```python
from build123d import *

# Parameters (mm, degrees)
SKETCH1_R           = 6
SKETCH1_R_2         = 2
BOSS_EXTRUDE1_DEPTH = 28.5
SKETCH2_R           = 2
SKETCH2_R_2         = 1
BOSS_EXTRUDE2_DEPTH = 3
SKETCH3_R           = 4
CUT_EXTRUDE1_DEPTH  = 23
SKETCH4_W           = 13
SKETCH4_H           = 13
SKETCH4_W_2         = 10
SKETCH4_H_2         = 10
CUT_EXTRUDE2_DEPTH  = 35.503622998
CUT_EXTRUDE5_DEPTH  = 33.003091855
SKETCH9_W           = 5
SKETCH9_H           = 4.708815116
CUT_EXTRUDE6_DEPTH  = 36.548469223
CUT_EXTRUDE7_DEPTH  = 35.412176554
SKETCH11_R          = 1.5
CUT_EXTRUDE8_DEPTH  = 32.929610206
FILLET1_R           = 2


with BuildPart() as part:
    # Sketch1 → Boss-Extrude1 (new body)
    with BuildSketch(Plane(origin=(0, 0, 0), x_dir=(1, 0, 0), z_dir=(0, 1, 0))):
        with Locations(Location((0, 0, 0), (0, 0, 90))):
            Circle(SKETCH1_R)
        with Locations(Location((0, 0, 0), (0, 0, 90))):
            Circle(SKETCH1_R_2, mode=Mode.SUBTRACT)
    extrude(amount=BOSS_EXTRUDE1_DEPTH)

    # Sketch2 → Boss-Extrude2 (add)
    with BuildSketch(Plane(origin=(0, -3, 0), x_dir=(-1, 0, 0), z_dir=(0, -1, 0))):
        with BuildLine():
            Line((-1.458956227, -17.348492079), (-5.300462758, -1.266089585))
            ThreePointArc((-5.300462758, -1.266089585), (0, 5.449576891), (5.300462758, -1.266089585))
            Line((5.300462758, -1.266089585), (1.458956227, -17.348492079))
            ThreePointArc((1.458956227, -17.348492079), (0, -18.5), (-1.458956227, -17.348492079))
        make_face()
        with Locations(Location((0, 0, 0), (0, 0, 90))):
            Circle(SKETCH2_R, mode=Mode.SUBTRACT)
        with Locations(Location((0, -17, 0), (0, 0, 90))):
            Circle(SKETCH2_R_2, mode=Mode.SUBTRACT)
    extrude(amount=-BOSS_EXTRUDE2_DEPTH)

    # Sketch3 → Cut-Extrude1 (cut)
    with BuildSketch(Plane(origin=(0, 28.5, 0), x_dir=(1, 0, 0), z_dir=(0, 1, 0))):
        with Locations(Location((0, 0, 0), (0, 0, 270))):
            Circle(SKETCH3_R)
    extrude(amount=-CUT_EXTRUDE1_DEPTH, mode=Mode.SUBTRACT)

    # Sketch4 → Cut-Extrude2 (cut, through all)
    with BuildSketch(Plane(origin=(0, 0, 0), x_dir=(1, 0, 0), z_dir=(0, 1, 0))):
        Rectangle(SKETCH4_W, SKETCH4_H)
        Rectangle(SKETCH4_W_2, SKETCH4_H_2, mode=Mode.SUBTRACT)
    extrude(amount=CUT_EXTRUDE2_DEPTH, mode=Mode.SUBTRACT)

    # Sketch8 → Cut-Extrude5 (cut, through all)
    with BuildSketch(Plane.XY.offset(5)):
        with BuildLine():
            Line((-5, 23.791184884), (-6.441511966, 23.791184884))
            Line((-6.441511966, 23.791184884), (-6.441511966, 29.385647876))
            Line((-6.441511966, 29.385647876), (5.988439259, 29.385647876))
            Line((5.988439259, 29.385647876), (5.988439259, 23.791184884))
            Line((5.988439259, 23.791184884), (5, 23.791184884))
            ThreePointArc((5, 23.791184884), (0, 28.5), (-5, 23.791184884))
        make_face()
    extrude(amount=-CUT_EXTRUDE5_DEPTH, mode=Mode.SUBTRACT)

    # Sketch9 → Cut-Extrude6 (cut, through all)
    with BuildSketch(Plane.ZY.offset(5)):
        with Locations((0, 26.145592442)):
            Rectangle(SKETCH9_W, SKETCH9_H)
        with BuildLine():
            Line((2.5, 23.791184884), (-2.5, 23.791184884))
            Line((-2.5, 23.791184884), (-2.5, 13.5))
            ThreePointArc((-2.5, 13.5), (0, 11), (2.5, 13.5))
            Line((2.5, 13.5), (2.5, 23.791184884))
        make_face()
    extrude(amount=-CUT_EXTRUDE6_DEPTH, mode=Mode.SUBTRACT)

    # Sketch10 → Cut-Extrude7 (cut, through all)
    with BuildSketch(Plane(origin=(0, 0, 0), x_dir=(1, 0, 0), z_dir=(0, 1, 0))):
        Polygon((-5, 3.31662479), (-5, -3.31662479), (-6.387377767, -3.31662479), (-6.387377767, 5), (-6.387377767, 6.820918536), (6.983329281, 6.820918536), (6.983329281, -3.31662479), (5, -3.31662479), (5, 5), (-5, 5), align=None)
    extrude(amount=-CUT_EXTRUDE7_DEPTH, mode=Mode.SUBTRACT)

    # Sketch11 → Cut-Extrude8 (cut, through all)
    with BuildSketch(Plane.XY.offset(5)):
        with Locations((0, 23)):
            Circle(SKETCH11_R)
    extrude(amount=-CUT_EXTRUDE8_DEPTH, mode=Mode.SUBTRACT)

    # Fillet1
    # the kernel refuses this fillet: 2 mm, written as the material it adds along each edge
    with BuildSketch(Plane(origin=(0, 0, 0), x_dir=(0.9752052541729319, 0, 0.22130230959822164), z_dir=(-0.22130230959822164, 0, 0.9752052541729319))) as fillet1_piece_1_section:
        with BuildLine():
            CenterArc((7.449576891, -1.377942973), FILLET1_R, 136.451251834, 43.548748166)
            Line((5.449576891, -1.377942973), (5.409576891, -1.377942973))
            Line((5.409576891, -1.377942973), (5.409576891, 0))
            Line((5.409576891, 0), (5.449576891, 0.04))
            ThreePointArc((5.449576891, 0.04), (5.724788445, 0.04), (5.971008462, 0.027558859))
            Line((5.971008462, 0.027558859), (6, 0))
        make_face()
    fillet1_piece_1 = revolve(axis=Axis((0, 0, 0), (0, 1, 0)), revolution_arc=115.571070831, mode=Mode.PRIVATE)
    fillet1_piece_1 = split(fillet1_piece_1, bisect_by=Plane(origin=(5, -0.397015398, -3.862769036), z_dir=(-1, 0, 0)), keep=Keep.TOP, mode=Mode.PRIVATE)
    fillet1_piece_1 = split(fillet1_piece_1, bisect_by=Plane(origin=(3.862770037, -0.397015398, -5), z_dir=(0, 0, 1)), keep=Keep.TOP, mode=Mode.PRIVATE)
    add(fillet1_piece_1)
    with BuildSketch(Plane(origin=(0, 0, 0), x_dir=(0.221302309598303, 0, -0.9752052541729136), z_dir=(0.9752052541729136, 0, 0.221302309598303))) as fillet1_piece_2_section:
        with BuildLine():
            CenterArc((7.449576891, -1.377942973), FILLET1_R, 136.451251834, 43.548748166)
            Line((6, 0), (5.971008462, 0.027558859))
            ThreePointArc((5.971008462, 0.027558859), (5.724788445, 0.04), (5.449576891, 0.04))
            Line((5.449576891, 0.04), (5.409576891, 0))
            Line((5.409576891, 0), (5.409576891, -1.377942973))
            Line((5.409576891, -1.377942973), (5.449576891, -1.377942973))
        make_face()
    fillet1_piece_2 = revolve(axis=Axis((0, 0, 0), (0, 1, 0)), revolution_arc=115.571070831, mode=Mode.PRIVATE)
    fillet1_piece_2 = split(fillet1_piece_2, bisect_by=Plane(origin=(-3.862770028, -0.397015251, -5), z_dir=(0, 0, 1)), keep=Keep.TOP, mode=Mode.PRIVATE)
    fillet1_piece_2 = split(fillet1_piece_2, bisect_by=Plane(origin=(-5, -0.397015251, -3.862769283), z_dir=(1, 0, 0)), keep=Keep.TOP, mode=Mode.PRIVATE)
    add(fillet1_piece_2)


solid = part.part
```
Can you work these out from the model? Positions are in its coordinate system, mm. A direction names the side the tool comes from. Give positions to 0.01 mm unless a question says otherwise; leave off trailing zeros. Write each loop counter-clockwise with the first axis right and the second up, starting at its lowest first coordinate (ties: lowest second). Pieces come first, ordered by that corner, then holes. Notation, with made-up numbers: (12.25, -3.75) -> (59.25, -3.75) arc R21 ccw to (59.25, 28.25) -> close; hole circle Ø1 at (79, -39.75). An arc over 180 degrees is marked (long way). Write item = value, one per line.
(1) Suppose I cut it at A-A on x = 0. Write out the boundary of the cut face in (y, z).
Worked out:
outline = (-3, -5) -> (21.5, -5) -> (21.5, -4) -> (5.5, -4) -> (5.5, -2) -> (-3, -2) -> close; (-3, 2) -> (5.5, 2) -> (5.5, 4) -> (21.5, 4) -> (21.5, 5) -> (0, 5) -> (0, 16) -> (-3, 16) -> close; (-3, 18) -> (0, 18) -> (0, 18.5) -> (-3, 18.5) -> close; (24.5, -5) -> (28.5, -5) -> (28.5, -4) -> (24.5, -4) -> close; (24.5, 4) -> (28.5, 4) -> (28.5, 5) -> (24.5, 5) -> close
(2) Suppose I cut it at C-C on y = 23. Write out the boundary of the cut face in (x, z).
Worked out:
outline = (-5, -3.32) arc R6 ccw to (-3.32, -5) -> (-1.5, -5) -> (-1.5, -3.71) arc R4 cw to (-3.12, -2.5) -> (-5, -2.5) -> close; (-5, 2.5) -> (-3.12, 2.5) arc R4 cw to (-1.5, 3.71) -> (-1.5, 5) -> (-3.32, 5) arc R6 ccw to (-5, 3.32) -> close; (1.5, -5) -> (3.32, -5) arc R6 ccw to (5, -3.32) -> (5, -2.5) -> (3.12, -2.5) arc R4 cw to (1.5, -3.71) -> close; (1.5, 3.71) arc R4 cw to (3.12, 2.5) -> (5, 2.5) -> (5, 3.32) arc R6 ccw to (3.32, 5) -> (1.5, 5) -> close
(3) Suppose I cut it at D-D on z = 0. Write out the boundary of the cut face in (x, y).
Worked out:
outline = (-5, -3) -> (-2, -3) -> (-2, 5.5) -> (-4, 5.5) -> (-4, 11) -> (-5, 11) -> close; (2, -3) -> (5, -3) -> (5, 11) -> (4, 11) -> (4, 5.5) -> (2, 5.5) -> close
(4) For faces 1 (the face through (4, 20, 2.5)), 2 (the face through (0, 14, 5)), 3 (the face through (-4.254, 13.432, 4.231)), 4 (the face through (3.874, -2.2, -3.833)), which set-ups out of +Z, -Z, +X, -X, +Y, -Y let a thin tool reach every point of the face, with its end or its side?
Worked out:
face_1 = +X, -X, +Y
face_2 = +Z, +X, -X, +Y
face_3 = +Z, -X, +Y
face_4 = -Z, +X, -Y
(5) I'm going to push flat-ended pins straight in: P1, Ø1.5, axis at x = -3.5, y = 6, coming from the +Z side; P2, Ø2, axis at x = -4.5, y = 19.5, coming from the -Z side; P3, Ø3, axis at x = 2, z = 12.5, coming from the +Y side. Where does each tip first touch, or does it pass through?
Worked out:
P1 = 5
P2 = -4.87
P3 = 0
(6) Thinking about a two-plate mould opening in Z: for faces 5 (the face through (4, 21, -2.5)), 6 (the face through (-5, 7, 0)), 7 (the face through (4.231, 13.432, 4.254)), which applies, released by +Z, released by -Z, zero draft, split by the parting line, or undercut?
Worked out:
face_5 = undercut
face_6 = zero draft
face_7 = released by +Z
(7) I need wall thicknesses on probe 1 along Z at (x, y) = (0, 19); probe 2 along Y at (x, z) = (0, -4.5); probe 3 along Z at (x, y) = (-3.25, 23.5). Which ranges of each line are inside material? Lowest first, please. Write a range as from..to.
Worked out:
probe_1 = -5..-4, 4..5
probe_2 = -3..21.5, 24.5..28.5
probe_3 = -5..-2.5, 2.5..5
(8) Suppose I cut it at B-B on y = 6. Write out the boundary of the cut face in (x, z).
Worked out:
outline = (-5, -3.32) arc R6 ccw to (-3.32, -5) -> (3.32, -5) arc R6 ccw to (5, -3.32) -> (5, 3.32) arc R6 ccw to (3.32, 5) -> (-3.32, 5) arc R6 ccw to (-5, 3.32) -> close; hole circle Ø8 at (0, 0)
